Autodesk Fusion 360 part; units mm, degrees
sketch "Boceto1" plane through (0, 0, 0) normal (0, 0, 1) x (1, 0, 0)
  circle A0 centre (0, 0) radius 1.575
  line L0 (0, 0) -> (12.5, 0)
  line L1 (12.5, 0) -> (12.5, 10)
  line L2 (12.5, 0) -> (12.5, -25)
  line L3 (12.5, 10) -> (-4.5, 10)
  line L4 (-4.5, 10) -> (-4.5, -35)
  line L5 (-4.5, -35) -> (12.5, -35)
  line L6 (12.5, -35) -> (12.5, 10)
  line L7 (12.5, -25) -> (0, -25)
  circle A1 centre (0, -25) radius 1.575
  line L8 (12.5, 10) -> (13.7, 10)
  line L9 (13.7, 10) -> (13.7, 8)
  line L10 (13.7, 8) -> (12.5, 8)
  line L11 (12.5, 8) -> (12.5, 10)
  line L12 (13.7, 5.4706) -> (12.5, 5.4706)
  line L13 (13.7, 7.4706) -> (13.7, 5.4706)
  line L14 (12.5, 7.4706) -> (13.7, 7.4706)
  line L15 (12.5, 5.4706) -> (12.5, 7.4706)
  line L16 (13.7, 2.9412) -> (12.5, 2.9412)
  line L17 (13.7, 4.9412) -> (13.7, 2.9412)
  line L18 (12.5, 4.9412) -> (13.7, 4.9412)
  line L19 (12.5, 2.9412) -> (12.5, 4.9412)
  line L20 (13.7, 0.4118) -> (12.5, 0.4118)
  line L21 (13.7, 2.4118) -> (13.7, 0.4118)
  line L22 (12.5, 2.4118) -> (13.7, 2.4118)
  line L23 (12.5, 0.4118) -> (12.5, 2.4118)
  line L24 (13.7, -2.1176) -> (12.5, -2.1176)
  line L25 (13.7, -0.1176) -> (13.7, -2.1176)
  line L26 (12.5, -0.1176) -> (13.7, -0.1176)
  line L27 (12.5, -2.1176) -> (12.5, -0.1176)
  line L28 (13.7, -4.6471) -> (12.5, -4.6471)
  line L29 (13.7, -2.6471) -> (13.7, -4.6471)
  line L30 (12.5, -2.6471) -> (13.7, -2.6471)
  line L31 (12.5, -4.6471) -> (12.5, -2.6471)
  line L32 (13.7, -7.1765) -> (12.5, -7.1765)
  line L33 (13.7, -5.1765) -> (13.7, -7.1765)
  line L34 (12.5, -5.1765) -> (13.7, -5.1765)
  line L35 (12.5, -7.1765) -> (12.5, -5.1765)
  line L36 (13.7, -9.7059) -> (12.5, -9.7059)
  line L37 (13.7, -7.7059) -> (13.7, -9.7059)
  line L38 (12.5, -7.7059) -> (13.7, -7.7059)
  line L39 (12.5, -9.7059) -> (12.5, -7.7059)
  line L40 (13.7, -12.2353) -> (12.5, -12.2353)
  line L41 (13.7, -10.2353) -> (13.7, -12.2353)
  line L42 (12.5, -10.2353) -> (13.7, -10.2353)
  line L43 (12.5, -12.2353) -> (12.5, -10.2353)
  line L44 (13.7, -14.7647) -> (12.5, -14.7647)
  line L45 (13.7, -12.7647) -> (13.7, -14.7647)
  line L46 (12.5, -12.7647) -> (13.7, -12.7647)
  line L47 (12.5, -14.7647) -> (12.5, -12.7647)
  line L48 (13.7, -17.2941) -> (12.5, -17.2941)
  line L49 (13.7, -15.2941) -> (13.7, -17.2941)
  line L50 (12.5, -15.2941) -> (13.7, -15.2941)
  line L51 (12.5, -17.2941) -> (12.5, -15.2941)
  line L52 (13.7, -19.8235) -> (12.5, -19.8235)
  line L53 (13.7, -17.8235) -> (13.7, -19.8235)
  line L54 (12.5, -17.8235) -> (13.7, -17.8235)
  line L55 (12.5, -19.8235) -> (12.5, -17.8235)
  line L56 (13.7, -22.3529) -> (12.5, -22.3529)
  line L57 (13.7, -20.3529) -> (13.7, -22.3529)
  line L58 (12.5, -20.3529) -> (13.7, -20.3529)
  line L59 (12.5, -22.3529) -> (12.5, -20.3529)
  line L60 (13.7, -24.8824) -> (12.5, -24.8824)
  line L61 (13.7, -22.8824) -> (13.7, -24.8824)
  line L62 (12.5, -22.8824) -> (13.7, -22.8824)
  line L63 (12.5, -24.8824) -> (12.5, -22.8824)
  line L64 (13.7, -27.4118) -> (12.5, -27.4118)
  line L65 (13.7, -25.4118) -> (13.7, -27.4118)
  line L66 (12.5, -25.4118) -> (13.7, -25.4118)
  line L67 (12.5, -27.4118) -> (12.5, -25.4118)
  line L68 (13.7, -29.9412) -> (12.5, -29.9412)
  line L69 (13.7, -27.9412) -> (13.7, -29.9412)
  line L70 (12.5, -27.9412) -> (13.7, -27.9412)
  line L71 (12.5, -29.9412) -> (12.5, -27.9412)
  line L72 (13.7, -32.4706) -> (12.5, -32.4706)
  line L73 (13.7, -30.4706) -> (13.7, -32.4706)
  line L74 (12.5, -30.4706) -> (13.7, -30.4706)
  line L75 (12.5, -32.4706) -> (12.5, -30.4706)
  line L76 (13.7, -35) -> (12.5, -35)
  line L77 (13.7, -33) -> (13.7, -35)
  line L78 (12.5, -33) -> (13.7, -33)
  line L79 (12.5, -35) -> (12.5, -33)
  dimension "d1" = 3.15
  dimension "d2" = 12.5
  dimension "d3" = 10
  dimension "d4" = 25
  dimension "d5" = 17
  dimension "d6" = 45
  dimension "d7" = 12.5
  dimension "d8" = 3.15
  dimension "d9" = 1.2
  dimension "d10" = 2
  dimension "d13" = 0
  dimension "d14" = -43
extrude "Extruir1" add sketch "Boceto1" along normal blind 3 makes body 1
copy_body "Cuerpo - > Comp.1" bodies 1 removing the originals makes body 2 in component "Cortina de Lamas"
extrude "Extruir1'" add sketch "Boceto1" against normal blind 75 contours L1 L6 L20 L21 L22 L23 | L2 L6 L24 L25 L26 L27 | L1 L6 L16 L17 L18 L19 | L2 L6 L28 L29 L30 L31 | L1 L6 L12 L13 L14 L15 | L2 L6 L32 L33 L34 L35 | L1 L6 L8 L9 L10 L11 | L2 L6 L36 L37 L38 L39 | L2 L6 L40 L41 L42 L43 | L6 L76 L77 L78 L79 | L2 L6 L44 L45 L46 L47 | L6 L72 L73 L74 L75 | L2 L6 L48 L49 L50 L51 | L6 L68 L69 L70 L71 | L2 L6 L52 L53 L54 L55 | L6 L64 L65 L66 L67 | L2 L6 L56 L57 L58 L59 | L2 L6 L60 L61 L62 L63 bodies 2 in component "Cortina de Lamas"
fillet "Empalme1" radius 8 2 edges at (-4.5, 10, 1.5) (-4.5, -35, 1.5) on bodies 2 in component "Cortina de Lamas"
component "Cortina de Lamas" placed x (1, 0, 0) y (0, 1, 0) z (0, 0, 1) at (0, 0, 0)
For this review, take the finished solid that the model builds, in its own axes (mm). A direction names the side the tool comes from. Round coordinates to 2 decimals unless told otherwise and drop trailing zeros. Loops run counter-clockwise (first coordinate to the right, second up) from the corner with the lowest first, then second, coordinate; pieces in that order, holes last. Notation, with made-up numbers: (-24.5, -18.75) - (11.5, -18.75) arc R22 cw to (11.5, 13.25) - close; hole circle Ø11 at (-17, 76). An arc over 180 degrees is marked (long way). One line per question, with ' | ' between items.
Q1. Take a section at A-A (x = 0). Give the boundary of the cut face in (y, z) (3 decimals), and give its area (3 significant figures).
Taken from the geometry:
outline: (-34.194, 0) - (-26.575, 0) - (-26.575, 3) - (-34.194, 3) - close; (-23.425, 0) - (-1.575, 0) - (-1.575, 3) - (-23.425, 3) - close; (1.575, 0) - (9.194, 0) - (9.194, 3) - (1.575, 3) - close | area: 111 mm²
Q2. Take a section at B-B (z = -64.5). State how many separate pieces and enclosed holes the cut face has, and give its area (3 significant figures).
Taken from the geometry:
separate pieces: 18 | enclosed holes: 0 | area: 43.2 mm²
Q3. Tool access review of faces 1 (the flat face through (13.7, -14, -37)), 2 (the flat face through (12.5, -6, -37)): name each direction out of +Z, -Z, +X, -X, +Y, -Y from which nothing blocks a thin tool from reaching the whole face with its end or side.
Taken from the geometry:
face 1: +Z, -Z, +X, +Y, -Y | face 2: -Z, -X, +Y, -Y
Q4. For line 1 along Y through (x, z) = (0, 1.1) (3 decimals); line 2 along Z through (x, y) = (2, 7.5); line 3 along X through (y, z) = (-25.5, -59), list the stretches that pass through material, from the lowest coordinate up. Write a range as [from, to].
Taken from the geometry:
line 1: y = [-34.194, -26.575], [-23.425, -1.575], [1.575, 9.194] | line 2: z = [0, 3] | line 3: x = [12.5, 13.7]
Q5. For pin 1 (3 mm diameter, centred on y = -29.5, z = -30, fed in from -X); pin 2 (0.6 mm diameter, centred on y = -25, z = 1.5, fed in from +X), all flat-tipped, find the tip position at first contact; note any pin that passes through.
Taken from the geometry:
pin 1: stops at x = 12.5 | pin 2: stops at x = 13.7
Q6. Take a section at C-C (y = -14). Give the boundary of the cut face in (x, z), and give its area (3 significant figures).
Taken from the geometry:
outline: (-4.5, 0) - (12.5, 0) - (12.5, -75) - (13.7, -75) - (13.7, 3) - (-4.5, 3) - close | area: 145 mm²
